Geometry: see drawing. Coordinates: mm, zero at the bounding-box minimum. A direction names the side the tool comes from. Give positions to 0.01 mm unless a question says otherwise; leave off trailing zeros. Order: outer loops, then holes, each group sorted by start corner. A loop starts at its lowest first (then second) coordinate and runs counter-clockwise, first axis right, second up. Notation, with made-up numbers: M 34.5,-20 L 82.5,-20 A20 ccw 82.5,-7 Z; hole C 33,70.25 d3. An arc over 180 degrees is marked long. Answer as a JSON object with one key per item and string values. Group by question number.
1. Section query A-A (y = 50). Output: boundary loops of the cut face in (x, z), plus the area to 3 significant figures.
2. Section query D-D (z = 37). Count the separate pieces of the cut face and the enclosed holes in it, plus the area to 3 significant figures.
3. Pull-direction query (Y, two-part tool) for the marked faces 1, 2, 3 and 4; classes: +Y half, -Y half, draft (parallel to the pull), parting line (faces both ways), or undercut.
4. Section query C-C (x = 40). Output: boundary loops of the cut face in (y, z).
5. Pin query (flat end, axial travel): P1, Ø10, axis at x = 42.5, z = 47, coming from the +Y side; P2, Ø6, axis at x = 25.5, z = 60, coming from the -Y side; P3, Ø16.5, axis at y = 32, z = 30, coming from the +X side; P4, Ø3.5, axis at y = 34.5, z = 21.5, coming from the +X side. Return the tip coordinate at first contact, or that it passes through.
6. Section query B-B (z = 21.5). Output: boundary loops of the cut face in (x, y), plus the area to 3 significant figures.
7. Set-up query: the marked faces 5, 6, 7 and 8. Return all of +Z, -Z, +X, -X, +Y, -Y with unobstructed straight access to the full face (end or side cutting, diameter ignored); none if empty.
8. Material intervals for L1, parallel to X at y = 6.6, z = 62; L2, parallel to Z at x = 40, y = 6; L3, parallel to Z at x = 40, y = 2, sorted ascending. Write a range as [from, to].
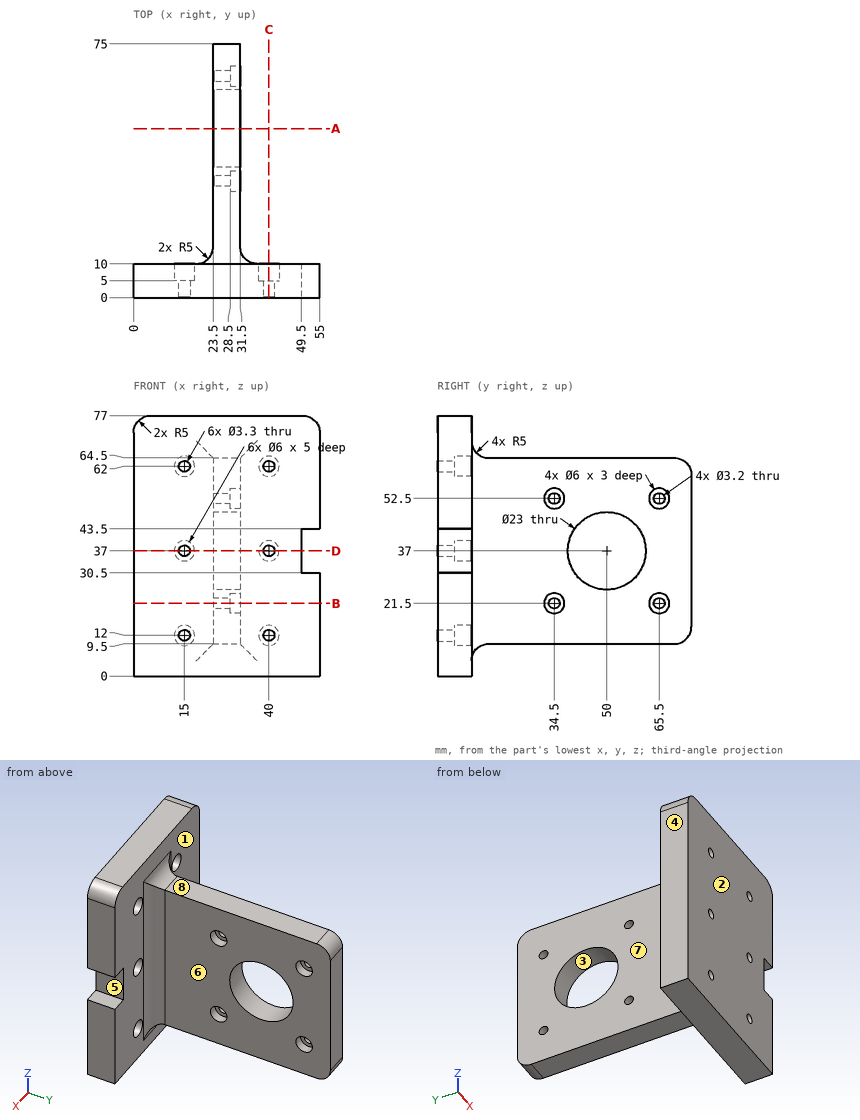
Answer sheet:
{
 "1": {"outline": "M 23.5,9.5 L 31.5,9.5 L 31.5,25.5 L 23.5,25.5 Z; M 23.5,48.5 L 31.5,48.5 L 31.5,64.5 L 23.5,64.5 Z", "area": "256 mm^2"},
 "2": {"separate pieces": "4", "enclosed holes": "0", "area": "749 mm^2"},
 "3": {"face 1": "+Y half", "face 2": "-Y half", "face 3": "undercut", "face 4": "draft"},
 "4": {"outline": "M 0,0 L 10,0 L 10,9 L 5,9 L 5,10.35 L 0,10.35 Z; M 0,13.65 L 5,13.65 L 5,15 L 10,15 L 10,34 L 5,34 L 5,35.35 L 0,35.35 Z; M 0,38.65 L 5,38.65 L 5,40 L 10,40 L 10,59 L 5,59 L 5,60.35 L 0,60.35 Z; M 0,63.65 L 5,63.65 L 5,65 L 10,65 L 10,77 L 0,77 Z"},
 "5": {"P1": "y = 10", "P2": "y = 0", "P3": "x = 31.5", "P4": "x = 28.5"},
 "6": {"outline": "M 0,0 L 55,0 L 55,10 L 36.5,10 A5 cw 31.5,15 L 31.5,31.5 L 28.5,31.5 L 28.5,32.9 L 23.5,32.9 L 23.5,15 A5 cw 18.5,10 L 0,10 Z; M 23.5,36.1 L 28.5,36.1 L 28.5,37.5 L 31.5,37.5 L 31.5,62.5 L 28.5,62.5 L 28.5,63.9 L 23.5,63.9 Z; M 23.5,67.1 L 28.5,67.1 L 28.5,68.5 L 31.5,68.5 L 31.5,75 L 23.5,75 Z", "area": "1,010 mm^2"},
 "7": {"face 5": "+X, +Y, -Y", "face 6": "+Z, -Z, +X, +Y", "face 7": "+Z, -Z, -X, +Y", "face 8": "+Z, +X, -X, +Y"},
 "8": {"L1": "[0, 12], [18, 37], [43, 55]", "L2": "[0, 9], [15, 34], [40, 59], [65, 77]", "L3": "[0, 10.35], [13.65, 35.35], [38.65, 60.35], [63.65, 77]"}
}
